Build history of the part. All positions in model axes, mm. Face numbers are marked on the shaded views. A direction names the side the tool comes from. Give positions to 0.01 mm unless a question says otherwise; leave off trailing zeros. Write each loop counter-clockwise with the first axis right and the second up, starting at its lowest first coordinate (ties: lowest second). Pieces come first, ordered by that corner, then holes. Notation, with made-up numbers: (-9.5, 0) -> (9.5, 0) arc R18 cw to (9.5, 29) -> close; hole circle Ø9 at (-21, 74.5). An arc over 180 degrees is marked (long way). One line per question, with ' | ' between items. Start each with the question number.
(1) Band-saw the part on A-A, the plane z = -2.5. Give the cut face in (x, y).
(2) Band-saw the part on D-D, the plane y = 28.5. Give the cut face in (x, z).
(3) Band-saw the part on B-B, the plane x = -10. Give the cut face in (y, z), and give its area (3 significant figures).
(4) Pin check, flat tips, straight feed: P1, Ø1.5, axis at y = 27.5, z = -3.5, coming from the -X side; P2, Ø2.5, axis at x = 8.5, z = -2, coming from the -Y side; P3, Ø2.5, axis at y = 27, z = -3, coming from the +X side. Stop position of each tip, or through.
(5) Band-saw the part on C-C, the plane y = 45.3. Give the cut face in (x, z), and give its area (3 significant figures).
(6) Pull direction X, two halves, no side cores. Call the marked faces 4, 5 and 6: released by +X, released by -X, zero draft, split by the parting line, or undercut.
(7) Tool access for the marked faces 1, 2 and 3: list every direction of +Z, -Z, +X, -X, +Y, -Y with a clear straight run to the whole face (end or side of a thin tool).
(8) Drill centre lines: probe 1 along X at (y, z) = (45.3, -2.8); probe 2 along X at (y, z) = (0.8, -2.5); probe 3 along X at (y, z) = (25.5, -3.45). Where is each one in solid material? Low to high. Write a range as from..to.
from build123d import *

# Parameters (mm, degrees)
SKETCH1_W               = 5
SKETCH1_H               = 3.288029927
SKETCH1_W_2             = 8
BOSS_EXTRUDE1_DEPTH     = 5
FILLET1_R               = 2
CUT_EXTRUDE1_DEPTH      = 56.795701159
CUT_EXTRUDE1_DEPTH_BACK = 56.795701159
SKETCH2_R               = 1.5
CUT_EXTRUDE2_DEPTH      = 59.463663929
CUT_EXTRUDE2_DEPTH_BACK = 59.463663929
SKETCH3_R               = 2.25
FILLET2_R               = 3


with BuildPart() as part:
    # Sketch1 → Boss-Extrude1 (new body)
    with BuildSketch(Plane.XY):
        Polygon((-5, 3.288029927), (0, 3.288029927), (0, 41), (20, 41), (20, 3.288029927), (25, 3.288029927), (25, 48), (-5, 48), align=None)
        with Locations((-2.5, 1.644014964)):
            Rectangle(SKETCH1_W, SKETCH1_H)
        with Locations((-9, 1.644014964)):
            Rectangle(SKETCH1_W_2, SKETCH1_H)
        with Locations((22.5, 1.644014964)):
            Rectangle(SKETCH1_W, SKETCH1_H)
        with Locations((29, 1.644014964)):
            Rectangle(SKETCH1_W_2, SKETCH1_H)
    extrude(amount=-BOSS_EXTRUDE1_DEPTH)

    # Fillet1
    fillet1_edges = [part.edges().sort_by_distance(p)[0] for p in [
        (-5, 48, -2.5),
        (25, 48, -2.5),
    ]]
    fillet(fillet1_edges, radius=FILLET1_R)

    # Sketch2 → Cut-Extrude1 (cut, two sides: drawn at the far end of the back side and taken through both)
    with BuildSketch(Plane(origin=(0, 3.288029927, 0), x_dir=(1, 0, 0), z_dir=(0, 1, 0)).offset(-CUT_EXTRUDE1_DEPTH_BACK)):
        with Locations(Location((-10, 2.5, 0), (0, 0, 180))):
            Circle(SKETCH2_R)
        with Locations(Location((30, 2.5, 0), (0, 0, 180))):
            Circle(SKETCH2_R)
    extrude(amount=CUT_EXTRUDE1_DEPTH + CUT_EXTRUDE1_DEPTH_BACK, mode=Mode.SUBTRACT)

    # Sketch3 → Cut-Extrude2 (cut, two sides: drawn at the far end of the back side and taken through both)
    with BuildSketch(Plane.XY.offset(-CUT_EXTRUDE2_DEPTH_BACK)):
        with Locations((14.513536336, 45.3)):
            Circle(SKETCH3_R)
        with Locations((5.486463664, 45.3)):
            Circle(SKETCH3_R)
    extrude(amount=CUT_EXTRUDE2_DEPTH + CUT_EXTRUDE2_DEPTH_BACK, mode=Mode.SUBTRACT)

    # Fillet2
    fillet2_edges = [part.edges().sort_by_distance(p)[0] for p in [
        (25, 3.288029927, -2.5),
        (-5, 3.288029927, -2.5),
    ]]
    fillet(fillet2_edges, radius=FILLET2_R)


solid = part.part
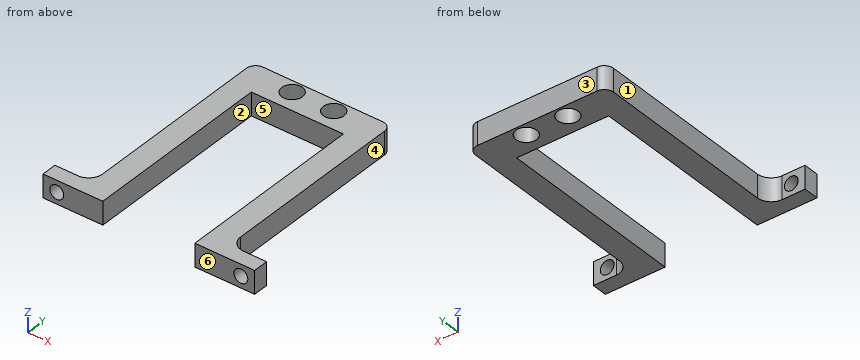
Results:
1) outline: (-13, 0) -> (-11.5, 0) -> (-11.5, 3.29) -> (-13, 3.29) -> close; (-8.5, 0) -> (0, 0) -> (0, 41) -> (20, 41) -> (20, 0) -> (28.5, 0) -> (28.5, 3.29) -> (28, 3.29) arc R3 cw to (25, 6.29) -> (25, 46) arc R2 ccw to (23, 48) -> (-3, 48) arc R2 ccw to (-5, 46) -> (-5, 6.29) arc R3 cw to (-8, 3.29) -> (-8.5, 3.29) -> close; (31.5, 0) -> (33, 0) -> (33, 3.29) -> (31.5, 3.29) -> close; hole circle Ø4.5 at (5.49, 45.3); hole circle Ø4.5 at (14.51, 45.3)
2) outline: (-5, -5) -> (0, -5) -> (0, 0) -> (-5, 0) -> close; (20, -5) -> (25, -5) -> (25, 0) -> (20, 0) -> close
3) outline: (0, -5) -> (3.29, -5) -> (3.29, -4) -> (0, -4) -> close; (0, -1) -> (3.29, -1) -> (3.29, 0) -> (0, 0) -> close | area: 6.58 mm²
4) P1: stops at x = -5 | P2: stops at y = 41 | P3: stops at x = 25
5) outline: (-5, -5) -> (3.24, -5) -> (3.24, 0) -> (-5, 0) -> close; (7.74, -5) -> (12.26, -5) -> (12.26, 0) -> (7.74, 0) -> close; (16.76, -5) -> (25, -5) -> (25, 0) -> (16.76, 0) -> close | area: 105 mm²
6) face 4: released by +X | face 5: undercut | face 6: zero draft
7) face 1: +Z, -Z, -X, +Y | face 2: +Z, -Z, -Y | face 3: +Z, -Z, +X, -X, +Y
8) probe 1: x = -5..3.24, 7.74..12.26, 16.76..25 | probe 2: x = -13..-11.5, -8.5..0, 20..28.5, 31.5..33 | probe 3: x = -5..0, 20..25
